CAD build for the part. Positions are in the model's coordinates, mm. A direction names the side the tool comes from. Coordinates: 2 decimals unless noted, no trailing zeros. Loops run counter-clockwise (first coordinate to the right, second up) from the corner with the lowest first, then second, coordinate; pieces in that order, holes last. Notation, with made-up numbers: (-36, -31.5) -> (-22, -31.5) arc R19 cw to (-22, 1.5) -> close; hole circle Ø6 at (-9.5, -35.5). An arc over 180 degrees is marked (long way). Return JSON: item names as keys, results as strings. Group by question number.
(1) Saw through at B-B on z = -173. Write the cut outline in (x, y), then the cut area to 3 significant figures.
(2) Saw through at C-C on x = 372.5. Write the cut outline in (y, z).
(3) Probe L1, parallel to Z at x = 19.5, y = -15; L2, parallel to Y at x = 480, z = -5; L3, parallel to X at y = -26.5, z = -97.5. List the from-to ranges inside material, lowest first.
(4) Saw through at A-A on y = -24. Write the cut outline in (x, z).
(5) Saw through at D-D on x = 429. Write the cut outline in (y, z), then the cut area to 3 significant figures.
(6) Flat gauge pins, fed straight in: pin 1 Ø5.5 at (y, z) = (-15, -160) entering from -X; pin 2 Ø5 at (y, z) = (-25.5, -247) entering from +X; pin 3 Ø11.5 at (y, z) = (-15, -50) entering from +X. Where does each tip first touch, or does it go through?
(7) Mould opens along Z. For faces 4 (the face through (0, -15, -148)), 5 (the face through (221.703, -14.79, -145.703)), 6 (the face through (15, -15, -300)), 7 (the face through (251, -15, 0)) say: pulls with the +Z half, pulls with the -Z half, needs draft (parallel to the pull), parting line crosses it, or undercut.
(8) Tool access for faces 1 (the face through (30, -15, -149)), 2 (the face through (483, -11, -30)), 3 (the face through (15.21, -12.635, -156.29)): list every direction of +Z, -Z, +X, -X, +Y, -Y with a clear straight run to the whole face (end or side of a thin tool).
```python
from build123d import *

# Parameters (mm, degrees)
F1_DEPTH = 30
F3_D     = 8.8
F3_DEPTH = 30
F3_TIP   = 2.6437867237
F5_D     = 8.8
F5_DEPTH = 30
F5_TIP   = 2.6437867237


with BuildPart() as f1:
    # F0 (on Front) → F1 (new body)
    with BuildSketch(Plane.XZ):
        Polygon((495, 0), (0, 0), (0, -300), (30, -300), (465, -30), (495, -30), align=None)
        Polygon((30, -264.6909348292), (30, -30), (408.1131727804, -30), align=None, mode=Mode.SUBTRACT)
    extrude(amount=F1_DEPTH)

    # F3
    with Locations(Plane(origin=(0, 0, 0), x_dir=(0, -1, 0), z_dir=(-1, 0, 0))):
        with Locations((15, -50), (15, -160)):
            Hole(F3_D / 2, depth=F3_DEPTH)
            with Locations((0, 0, -(F3_DEPTH + F3_TIP / 2))):  # 118° drill point
                Cone(0, F3_D / 2, F3_TIP, mode=Mode.SUBTRACT)

    # F5
    with Locations(Plane.XY):
        with Locations((480, -15), (50, -15)):
            Hole(F5_D / 2, depth=F5_DEPTH)
            with Locations((0, 0, -(F5_DEPTH + F5_TIP / 2))):  # 118° drill point
                Cone(0, F5_D / 2, F5_TIP, mode=Mode.SUBTRACT)


solid = f1.part
```
Geometry results:
{
 "1": {"outline": "(0, -30) -> (30, -30) -> (30, 0) -> (0, 0) -> close; (177.72, -30) -> (234.61, -30) -> (234.61, 0) -> (177.72, 0) -> close", "area": "2,610 mm²"},
 "2": {"outline": "(-30, -87.41) -> (0, -87.41) -> (0, -52.1) -> (-30, -52.1) -> close; (-30, -30) -> (0, -30) -> (0, 0) -> (-30, 0) -> close"},
 "3": {"L1": "-300 to -164.4, -155.6 to -54.4, -45.6 to 0", "L2": "-30 to -19.4, -10.6 to 0", "L3": "0 to 30, 299.36 to 356.25"},
 "4": {"outline": "(0, -300) -> (30, -300) -> (465, -30) -> (495, -30) -> (495, 0) -> (0, 0) -> close; hole (30, -264.69) -> (408.11, -30) -> (30, -30) -> close"},
 "5": {"outline": "(-30, -52.34) -> (0, -52.34) -> (0, 0) -> (-30, 0) -> close", "area": "1,570 mm²"},
 "6": {"pin 1": "x = 194.24", "pin 2": "x = 119.42", "pin 3": "x = 442.04"},
 "7": {"face 4": "needs draft", "face 5": "undercut", "face 6": "pulls with the -Z half", "face 7": "pulls with the +Z half"},
 "8": {"face 1": "+Y, -Y", "face 2": "-Z, +X, +Y, -Y", "face 3": "-X"}
}
